from build123d import *

# Parameters (mm, degrees)
F0_W     = 1000
F0_H     = 300
F1_DEPTH = 25
F2_W     = 275
F2_H     = 5
F3_DEPTH = 1000.001
F5_DEPTH = 300.001
F7_DEPTH = 300.001
F9_DEPTH = 5


with BuildPart() as f1:
    # F0 (on Top) → F1 (new body)
    with BuildSketch(Plane.XY):
        with Locations((514.9225434339, 4.54775244)):
            Rectangle(F0_W, F0_H)
    extrude(amount=F1_DEPTH)

    # F2 (on face) → F3 (cut, through all)
    with BuildSketch(Plane.YZ.offset(1014.9225434339)):
        with Locations((17.04775244, 12.5)):
            Rectangle(F2_W, F2_H)
    extrude(amount=-F3_DEPTH, mode=Mode.SUBTRACT)

    # F4 (on face) → F5 (cut, through all)
    with BuildSketch(Plane(origin=(0, 154.54775244, 0), x_dir=(-1, 0, 0), z_dir=(0, 1, 0))):
        with BuildLine():
            ThreePointArc((-992.1274558663, 15), (-1004.3292812217, 18.1666331145), (-1014.9225434339, 25))
            Line((-1014.9225434339, 25), (-1014.9225434339, 15))
            Line((-1014.9225434339, 15), (-992.1274558663, 15))
        make_face()
    extrude(amount=-F5_DEPTH, mode=Mode.SUBTRACT)

    # F6 (on face) → F7 (cut, through all)
    with BuildSketch(Plane(origin=(0, 154.54775244, 0), x_dir=(-1, 0, 0), z_dir=(0, 1, 0))):
        with BuildLine():
            ThreePointArc((-1014.9225434339, 0), (-1002.414847544, 6.8277253985), (-988.5225128069, 10))
            Line((-988.5225128069, 10), (-1014.9225434339, 10))
            Line((-1014.9225434339, 10), (-1014.9225434339, 0))
        make_face()
    extrude(amount=-F7_DEPTH, mode=Mode.SUBTRACT)

    # F8 (on face) → F9 (cut)
    with BuildSketch(Plane.XY.offset(15)):
        with BuildLine():
            ThreePointArc((992.1274558663, -120.45224756), (1008.3682439808, -128.5361604148), (1014.9225434339, -145.45224756))
            Line((1014.9225434339, -145.45224756), (1014.9225434339, -120.45224756))
            Line((1014.9225434339, -120.45224756), (992.1274558663, -120.45224756))
        make_face()
    extrude(amount=-F9_DEPTH, mode=Mode.SUBTRACT)


solid = f1.part
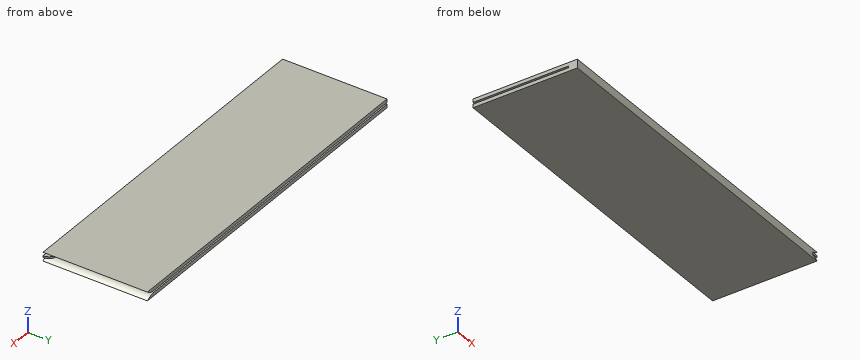
Part model, mm, in its own coordinate system. Coordinates: 2 decimals unless noted, no trailing zeros. Order: outer loops, then holes, each group sorted by start corner. A loop starts at its lowest first (then second) coordinate and runs counter-clockwise, first axis right, second up. Notation, with made-up numbers: (84, 81.25) - (120, 81.25) arc R18 cw to (120, 85.25) - close; hole circle Ø7 at (-10, 30). An arc over 180 degrees is marked (long way). Use CSV: the item, a comma, the result in double quotes.
Item 1: Saw through at A-A on y = 21. Give the cut face in (x, z).
Solved:
outline,"(14.92, 0) - (1014.92, 0) arc R51.95 ccw to (988.52, 10) - (14.92, 10) - close; (14.92, 15) - (992.13, 15) arc R39.69 ccw to (1014.92, 25) - (14.92, 25) - close"
Item 2: Saw through at B-B on x = 803. Give the cut face in (y, z), and give its area (4 significant figures).
Solved:
outline,"(-145.45, 0) - (154.55, 0) - (154.55, 10) - (-120.45, 10) - (-120.45, 15) - (154.55, 15) - (154.55, 25) - (-145.45, 25) - close"
area,"6,125 mm²"
Item 3: Probe probe 1 along Z at (x, y) = (691, -15.5); probe 2 along Y at (x, z) = (967, 13.5); probe 3 along X at (y, z) = (116, 23.25). List the from-to ranges inside material, lowest first.
Solved:
probe 1,"z = 0 to 10, 15 to 25"
probe 2,"y = -145.45 to -120.45"
probe 3,"x = 14.92 to 1012.84"
Item 4: Drop a flat-ended pin along its axis: P1, Ø4, axis at y = -17.5, z = 4, coming from the +X side. Give the stop position or say it passes through.
Solved:
P1,"stops at x = 1012.02"
